Autodesk Inventor part; units mm, degrees
ref_plane "YZ Plane" through (0, 0, 0) normal (1, 0, 0) x (0, 1, 0)
ref_plane "XZ Plane" through (0, 0, 0) normal (0, 1, 0) x (-1, 0, 0)
ref_plane "XY Plane" through (0, 0, 0) normal (0, 0, 1) x (1, 0, 0)
sketch "Sketch1" plane through (0, 0, 0) normal (0, 1, 0) x (-1, 0, 0)
  line L0 (-12.7, 12.7) -> (12.7, 12.7)
  line L1 (12.7, 12.7) -> (12.7, -12.7)
  line L2 (12.7, -12.7) -> (-12.7, -12.7)
  line L3 (-12.7, -12.7) -> (-12.7, 12.7)
  line L4 (-12.7, 12.7) -> (12.7, -12.7) construction
  line L5 (12.7, 12.7) -> (-12.7, -12.7) construction
  line L6 (14.9209, 3.2512) -> (10.4791, 3.2512)
  line L7 (10.4791, 3.2512) -> (10.4791, -3.2512)
  line L8 (10.4791, -3.2512) -> (14.9209, -3.2512)
  line L9 (14.9209, -3.2512) -> (14.9209, 3.2512)
  line L10 (14.9209, 3.2512) -> (10.4791, -3.2512) construction
  line L11 (10.4791, 3.2512) -> (14.9209, -3.2512) construction
  line L12 (12.7, 3.2512) -> (10.4902, 3.2512)
  line L13 (10.4902, 3.2512) -> (10.4902, 9.3687)
  line L14 (10.4902, 9.3687) -> (12.7, 9.3687)
  line L15 (12.7, 9.3687) -> (12.7, 3.2512)
  line L16 (-4.5426, 4.5426) -> (4.5426, 4.5426)
  line L17 (4.5426, 1.686) -> (4.5426, -1.686)
  line L18 (4.5426, -4.5426) -> (-4.5426, -4.5426)
  line L19 (-4.5426, -4.5426) -> (-4.5426, 4.5426)
  line L20 (-4.5426, 4.5426) -> (4.5426, -4.5426) construction
  line L21 (4.5426, 4.5426) -> (-4.5426, -4.5426) construction
  line L22 (12.7, 12.7) -> (-12.7, -12.7) construction
  line L23 (11.9293, 13.4707) -> (-13.4707, -11.9293)
  line L24 (5.4725, 3.9311) -> (13.4707, 11.9293)
  arc A0 (13.4707, 11.9293) -> (11.9293, 13.4707) centre (12.7, 12.7) ccw
  arc A1 (-13.4707, -11.9293) -> (-11.9293, -13.4707) centre (-12.7, -12.7) ccw
  line L25 (12.7, -12.7) -> (-12.7, 12.7) construction
  line L26 (11.9293, -13.4707) -> (-13.4707, 11.9293)
  line L27 (5.4725, -3.9311) -> (13.4707, -11.9293)
  arc A2 (11.9293, -13.4707) -> (13.4707, -11.9293) centre (12.7, -12.7) ccw
  arc A3 (-11.9293, 13.4707) -> (-13.4707, 11.9293) centre (-12.7, 12.7) ccw
  arc A4 (5.4725, 3.9311) -> (4.5426, 1.686) centre (7.7176, 1.686) ccw
  arc A5 (4.5426, -1.686) -> (5.4725, -3.9311) centre (7.7176, -1.686) ccw
  point P0 (0, 0)
  point P1 (12.7, 0)
  point P2 (0, 0)
  point P3 (0, 0)
  dimension "d0" = 25.4
  dimension "d1" = 25.4
  dimension "d2" = 6.5024
  dimension "d3" = 2.2098
  dimension "d4" = 3.175
sketch "Sketch2" plane through (0, 0, 0) normal (0, 1, 0) x (-1, 0, 0)
  line L0 (9.3228, 7.7741) -> (5.6047, 4.0154)
  line L1 (5.6047, 4.0154) -> (5.5129, 3.9226)
  line L2 (4.5951, 1.6897) -> (4.5951, 0)
  line L3 (9.7743, 7.9625) -> (9.7971, 7.9625)
  line L4 (10.4321, 7.3275) -> (10.4321, 3.1448)
  line L5 (10.4321, 3.1448) -> (13.3143, 3.1448)
  arc A0 (5.5129, 3.9226) -> (4.5951, 1.6897) centre (7.7701, 1.6897) ccw
  arc A1 (9.7743, 7.9625) -> (9.3228, 7.7741) centre (9.7743, 7.3275) ccw
  arc A2 (10.4321, 7.3275) -> (9.7971, 7.9625) centre (9.7971, 7.3275) ccw
  line L6 (13.3143, 3.1448) -> (13.3143, 7.9625)
  line L7 (13.3143, 7.9625) -> (12.6666, 9.6561)
  line L8 (12.6666, 9.6561) -> (12.6666, 10.8508)
  line L9 (12.6666, 10.8508) -> (14.9475, 10.8508)
  line L10 (14.9475, 10.8508) -> (16.328, 10.8508)
  line L11 (16.328, 10.8508) -> (23.2713, 3.1448)
  line L12 (23.2713, 3.1448) -> (23.2713, 0)
  line L13 (9.3228, -7.7741) -> (5.6047, -4.0154)
  line L14 (4.5951, -1.6897) -> (4.5951, 0)
  line L15 (10.4321, -7.3275) -> (10.4321, -3.1448)
  line L16 (10.4321, -3.1448) -> (13.3143, -3.1448)
  arc A3 (4.5951, -1.6897) -> (5.5129, -3.9226) centre (7.7701, -1.6897) ccw
  arc A4 (9.3228, -7.7741) -> (9.7743, -7.9625) centre (9.7743, -7.3275) ccw
  arc A5 (9.7971, -7.9625) -> (10.4321, -7.3275) centre (9.7971, -7.3275) ccw
  line L17 (13.3143, -3.1448) -> (13.3143, -7.9625)
  line L18 (13.3143, -7.9625) -> (12.6666, -9.6561)
  line L19 (12.6666, -9.6561) -> (12.6666, -10.8508)
  line L20 (12.6666, -10.8508) -> (14.9475, -10.8508)
  line L21 (14.9475, -10.8508) -> (16.328, -10.8508)
  line L22 (16.328, -10.8508) -> (23.2713, -3.1448)
  line L23 (23.2713, -3.1448) -> (23.2713, 0)
  line L24 (5.5129, -3.9226) -> (5.6047, -4.0154)
  line L25 (9.7971, -7.9625) -> (9.7743, -7.9625)
  point P0 (0, 0)
  point P1 (4.5951, 2.9948)
  dimension "d5" = 3.175
  dimension "d6" = 0.635
extrude "Extrusion1" add sketch "Sketch2" along normal blind 6.35
properties part number "sliding_t_nut_prototype01"
The model under review builds one solid part; all positions refer to its coordinate system, in mm. A direction names the side the tool comes from. Round coordinates to 2 decimals unless told otherwise and drop trailing zeros. Write each loop counter-clockwise with the first axis right and the second up, starting at its lowest first coordinate (ties: lowest second). Pieces come first, ordered by that corner, then holes. Notation, with made-up numbers: (14, 62) - (27, 62) arc R14 cw to (27, 66) - close; hole circle Ø10 at (67.25, 53.5). An arc over 180 degrees is marked (long way). One line per question, with ' | ' between items.
Item 1: Add section B-B, the plane x = -8.75. Give the boundary of the cut face in (y, z).
Resolved:
outline: (0, -7.2) - (6.35, -7.2) - (6.35, 7.2) - (0, 7.2) - close
Item 2: For P1, Ø3, axis at y = 0.5, z = -2, coming from the +X side; P2, Ø1, axis at y = 3.5, z = 10, coming from the +X side; P3, Ø1.4, axis at y = 4.5, z = 4.5, coming from the +X side; P4, Ø1.5, axis at y = 0.5, z = -6.5, coming from the +X side, all flat-tipped, find the tip position at first contact; note any pin that passes through.
Resolved:
P1: stops at x = -4.6 | P2: stops at x = -12.67 | P3: stops at x = -5.4 | P4: stops at x = -7.32
Item 3: To check wall thickness, follow probe 1 along X at (y, z) = (3.5, 5); probe 2 along Z at (x, y) = (-12.5, 5); probe 3 along Z at (x, y) = (-19.5, 5). State the ranges of each line that lie inside material, in increasing order.
Resolved:
probe 1: x = -21.6 to -13.31, -10.43 to -6.58 | probe 2: z = -3.14 to 3.14 | probe 3: z = -7.33 to 7.33
Item 4: For faces 5 (the face through (-12, 3, 3.145)), 6 (the face through (-12.667, 3, -10)), 7 (the face through (-12.995, 3.131, -8.797)), 8 (the face through (-12.667, 3, 10)), 9 (the face through (-10.432, 3, -5)), list the 3-axis set-ups (+Z, -Z, +X, -X, +Y, -Y) from which the entire face can be reached by the end or side of a thin tool; tool diameter is ignored.
Resolved:
face 5: +Y, -Y | face 6: -Z, +X, +Y, -Y | face 7: +X, +Y, -Y | face 8: +Z, +X, +Y, -Y | face 9: -Z, +Y, -Y
Item 5: Add section C-C, the plane z = 8.5. Give the boundary of the cut face in (x, y), then the cut area to 3 significant figures.
Resolved:
outline: (-18.45, 0) - (-13.11, 0) - (-13.11, 6.35) - (-18.45, 6.35) - close | area: 33.9 mm2
Item 6: The part is to be moulded in two halves that separate along Z. For faces 1 (the face through (-14, 0, 0)), 2 (the face through (-13.314, 3, 6)), 3 (the face through (-13.314, 3, -6)), 4 (the face through (-19.75, 3.13, -7.05)), say which applies: pulls with the +Z half, pulls with the -Z half, needs draft (parallel to the pull), parting line crosses it, or undercut.
Resolved:
face 1: needs draft | face 2: undercut | face 3: undercut | face 4: pulls with the -Z half
